from build123d import *

# Parameters (mm, degrees)
SKETCH1_R         = 7
EXTRUDE1_DEPTH    = 129
EXTRUDE2_START    = -46
SKETCH2_R         = 9
EXTRUDE2_DEPTH    = 4
EXTRUDE3_START    = 4
EXTRUDE3_DEPTH    = 126.626386203
SKETCH4_OUTSIDE_W = 46.298
SKETCH4_OUTSIDE_H = 46.298
SKETCH4_OUTSIDE_R = 6
EXTRUDE4_DEPTH    = 10
CHAMFER1_SIZE     = 0.3
SKETCH5_OUTSIDE_W = 46.298
SKETCH5_OUTSIDE_H = 46.298
SKETCH5_OUTSIDE_R = 6.8
EXTRUDE5_DEPTH    = 63
CHAMFER2_SIZE     = 0.3


with BuildPart() as part:
    # Sketch1 → Extrude1 (new body)
    with BuildSketch(Plane.XY):
        Circle(SKETCH1_R)
    extrude(amount=EXTRUDE1_DEPTH)

    # Sketch2 → Extrude2 (add)
    with BuildSketch(Plane.XY.offset(129).offset(EXTRUDE2_START)):
        Circle(SKETCH2_R)
    extrude(amount=EXTRUDE2_DEPTH)

    # Sketch3 → Extrude3 (cut, through all)
    with BuildSketch(Plane(origin=(0, 0, 0), x_dir=(0, 0, -1), z_dir=(1, 0, 0)).offset(EXTRUDE3_START)):
        with BuildLine():
            Line((-83, 2.5), (-63, 2.5))
            ThreePointArc((-63, 2.5), (-60.5, 0), (-63, -2.5))
            Line((-63, -2.5), (-83, -2.5))
            ThreePointArc((-83, -2.5), (-85.5, 0), (-83, 2.5))
        make_face()
    extrude(amount=EXTRUDE3_DEPTH, mode=Mode.SUBTRACT)

    # Sketch4 outside → Extrude4 (cut)
    with BuildSketch(Plane(origin=(0, 0, 0), x_dir=(-1, 0, 0), z_dir=(0, 0, -1))):
        Rectangle(SKETCH4_OUTSIDE_W, SKETCH4_OUTSIDE_H)
        Circle(SKETCH4_OUTSIDE_R, mode=Mode.SUBTRACT)
    extrude(amount=-EXTRUDE4_DEPTH, mode=Mode.SUBTRACT)

    # Chamfer1
    chamfer1_edges = [part.edges().sort_by_distance(p)[0] for p in [
        (6, 0, 0),
        (-7, 0, 129),
        (-9, 0, 87),
        (-9, 0, 83),
        (-7, 0, 10),
    ]]
    chamfer(chamfer1_edges, length=CHAMFER1_SIZE)

    # Sketch5 outside → Extrude5 (cut)
    with BuildSketch(Plane(origin=(0, 0, 0), x_dir=(-1, 0, 0), z_dir=(0, 0, -1))):
        Rectangle(SKETCH5_OUTSIDE_W, SKETCH5_OUTSIDE_H)
        with Locations(Location((0, 0, 0), (0, 0, 158.429421698))):
            Circle(SKETCH5_OUTSIDE_R, mode=Mode.SUBTRACT)
    extrude(amount=-EXTRUDE5_DEPTH, mode=Mode.SUBTRACT)

    # Chamfer2
    # the kernel refuses this chamfer: 0.3 mm, written as the material it takes off along each edge
    with BuildSketch(Plane(origin=(0, 0, 63), x_dir=(0.9678051111401075, -0.25170074861049596, 0), z_dir=(0.25170074861049596, 0.9678051111401075, 0))) as chamfer2_piece_1_section:
        Polygon((7, -CHAMFER2_SIZE), (7 - CHAMFER2_SIZE, 0), (7, 0), align=None)
    chamfer2_piece_1 = revolve(axis=Axis((0, 0, 63), (0, 0, -1)), revolution_arc=330.843646851, mode=Mode.PRIVATE)
    chamfer2_piece_1 = chamfer2_piece_1 - Plane(origin=(0, 0, 63.195747315), x_dir=(0.9299653972776295, 0.36764705882987936, 0), z_dir=(0, 0, -1)) * Cylinder(6.8, 28, mode=Mode.PRIVATE)
    add(chamfer2_piece_1, mode=Mode.SUBTRACT)


solid = part.part
Read the model definition and answer for the solid it produces. Units are mm, in the model's axes. A direction names the side the tool comes from. Coordinates: 2 decimals unless noted, no trailing zeros. Loops run counter-clockwise (first coordinate to the right, second up) from the corner with the lowest first, then second, coordinate; pieces in that order, holes last. Notation, with made-up numbers: (68, 61) -> (111, 61) arc R10 cw to (111, 71) -> close; hole circle Ø4 at (-5, 8). An arc over 180 degrees is marked (long way). Answer in a Markdown table with one row per item.
Item 1: For a pull along Z with two mould halves and no side action, classify faces 1 (the cylindrical face through (6.783, 0.485, 36.229)), 2 (the flat face through (-7, -3, 83)), 3 (the flat face through (0, 0, 129)), 4 (the cylindrical face through (5.4, 0.1, 60.5)) as released by +Z, released by -Z, zero draft, split by the parting line, or undercut.
Returned:
| item | result |
|---|---|
| face 1 | zero draft |
| face 2 | released by -Z |
| face 3 | released by +Z |
| face 4 | undercut |
Item 2: Straight lines are drawn through the part: line 1 along Z through (x, y) = (2.25, -7.25); line 2 along X through (y, z) = (-0.5, 67); line 3 along Y through (x, z) = (0.25, 37.5). For each, find the intervals that lie inside material, in ascending order. Write a range as [from, to].
Returned:
| item | result |
|---|---|
| line 1 | z = [83, 87] |
| line 2 | x = [-6.98, 4] |
| line 3 | y = [-6.8, 6.8] |
Item 3: A cutting plane is placed at C-C on z = 73. Determine the outline of the cut face in (x, y).
Returned:
| item | result |
|---|---|
| outline | (4, -2.5) -> (4, 2.5) -> (6.54, 2.5) arc R7 ccw (long way) to (6.54, -2.5) -> close |
Item 4: For faces 5 (the cylindrical face through (6.5, -0.1, 85.5)), 6 (the flat face through (2, -6, 10)), 7 (the flat face through (-6, 4, 87)), determine the directions among +Z, -Z, +X, -X, +Y, -Y from which every point of the face is accessible in a straight line to the end or side of a thin tool.
Returned:
| item | result |
|---|---|
| face 5 | +X |
| face 6 | -Z |
| face 7 | +Z |
Item 5: A cutting plane is placed at D-D on z = 114. Determine the outline of the cut face in (x, y), plus the area to 3 significant figures.
Returned:
| item | result |
|---|---|
| outline | circle Ø14 at (0, 0) |
| area | 154 mm^2 |
Item 6: Each of these flat-tipped pins is pushed along its axis until it touches: P1, Ø10, axis at x = 5, y = 7, coming from the -Z side; P2, Ø6, axis at y = -6, z = 40.5, coming from the +X side; P3, Ø6, axis at y = -2.5, z = 62, coming from the -X side; P4, Ø2, axis at x = -7, z = 60.5, coming from the -Y side. Where does it stop, or does it pass through?
Returned:
| item | result |
|---|---|
| P1 | stops at z = 0 |
| P2 | stops at x = 6.1 |
| P3 | stops at x = -7 |
| P4 | stops at y = -3.2 |
